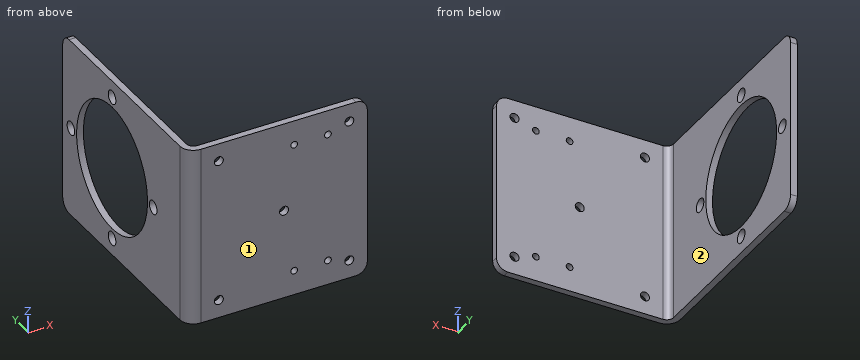
```python
from build123d import *

# Parameters (mm, degrees)
SKETCH1_W                        = 80
SKETCH1_H                        = 98.5
SKETCH1_R                        = 28
BASE_FLANGE1_DEPTH               = 3
F_6_0_6_DIAMETER_HOLE1_D         = 6
CIRPATTERN1_COUNT                = 4
SM_EDGE_FLANGE_1_STRIP_W         = 18
SM_EDGE_FLANGE_1_STRIP_H         = 3
SM_EDGE_FLANGE_1_STRIP_CUT_DEPTH = 80
SM_EDGE_FLANGE_1_DEPTH           = 80
FILLET1_R                        = 5
F_4_0_4_DIAMETER_HOLE4_D         = 4
F_3_0_3_DIAMETER_HOLE2_D         = 3


# Sheet-metal steps are written as plain solids
with BuildPart() as part:
    # Sketch1 → Base-Flange1 (new body)
    with BuildSketch(Plane(origin=(0, 0, 0), x_dir=(0, 0, -1), z_dir=(1, 0, 0))):
        with Locations((40, 49.25)):
            Rectangle(SKETCH1_W, SKETCH1_H)
        with Locations((40, 59.5)):
            Circle(SKETCH1_R, mode=Mode.SUBTRACT)
    extrude(amount=-BASE_FLANGE1_DEPTH)

    # Ø6.0 (6) Diameter Hole1 (through all)
    with Locations(Plane(origin=(0, 0, 0), x_dir=(0, 0, -1), z_dir=(1, 0, 0))):
        with Locations((40, 92)):
            f_6_0_6_diameter_hole1 = Hole(F_6_0_6_DIAMETER_HOLE1_D / 2)

    # CirPattern1: Ø6.0 (6) Diameter Hole1 ×4 about axis
    cirpattern1_axis = Axis((0, 59.5, -40), (1, 0, 0))
    for i in range(1, CIRPATTERN1_COUNT):
        add(f_6_0_6_diameter_hole1.rotate(cirpattern1_axis, i * 360 / CIRPATTERN1_COUNT), mode=Mode.SUBTRACT)

    # 邊線-凸緣1 strip (across the edge) → 邊線-凸緣1 strip cut (cut)
    with BuildSketch(Plane.YX):
        with Locations((-3, -1.5)):
            Rectangle(SM_EDGE_FLANGE_1_STRIP_W, SM_EDGE_FLANGE_1_STRIP_H)
    extrude(amount=SM_EDGE_FLANGE_1_STRIP_CUT_DEPTH, mode=Mode.SUBTRACT)

    # 邊線-凸緣1 section (across the edge) → 邊線-凸緣1 (add)
    with BuildSketch(Plane.YX):
        with BuildLine():
            Line((0, 3), (0, 77))
            Line((0, 77), (3, 77))
            Line((3, 77), (3, 3))
            ThreePointArc((3, 3), (3.878679656, 0.878679656), (6, 0))
            Line((6, 0), (6, -3))
            ThreePointArc((6, -3), (1.757359313, -1.242640687), (0, 3))
        make_face()
    extrude(amount=SM_EDGE_FLANGE_1_DEPTH)

    # Fillet1
    fillet1_edges = [part.edges().sort_by_distance(p)[0] for p in [
        (77, 1.5, 0),
        (77, 1.5, -80),
        (-1.5, 98.5, 0),
        (-1.5, 98.5, -80),
    ]]
    fillet(fillet1_edges, radius=FILLET1_R)

    # Ø4.0 (4) Diameter Hole4 (through all)
    with Locations(Plane(origin=(0, 3, 0), x_dir=(1, 0, 0), z_dir=(0, 1, 0))):
        with Locations((11, 8), (11, 72), (69, 72), (69, 8), (40, 40)):
            Hole(F_4_0_4_DIAMETER_HOLE4_D / 2)

    # Ø3.0 (3) Diameter Hole2 (through all)
    with Locations(Plane(origin=(0, 3, 0), x_dir=(1, 0, 0), z_dir=(0, 1, 0))):
        with Locations((44.5, 11), (59.5, 11)):
            f_3_0_3_diameter_hole2 = Hole(F_3_0_3_DIAMETER_HOLE2_D / 2)

    # Mirror1: Ø3.0 (3) Diameter Hole2 across plane
    add(f_3_0_3_diameter_hole2.mirror(Plane.XY.offset(-40)), mode=Mode.SUBTRACT)


solid = part.part
```
Check sheet for the modelled part. Datum: model origin and axes. Units: mm. Face numbers are marked on the shaded views. A direction names the side the tool comes from. Give positions to 0.01 mm unless a question says otherwise; leave off trailing zeros. Write each loop counter-clockwise with the first axis right and the second up, starting at its lowest first coordinate (ties: lowest second). Pieces come first, ordered by that corner, then holes. Notation, with made-up numbers: (44.5, -28.75) -> (98.5, -28.75) arc R19 ccw to (98.5, -24.75) -> close; hole circle Ø6 at (85.5, 10.25). An arc over 180 degrees is marked (long way). Use CSV: the item, a comma, the result in double quotes. Start each with the question number.
Q1. Cross-section at B-B on z = -40. Enter the section's corners in (x, y).
Q2. Cross-section at D-D on x = 11. Enter the section's corners in (y, z), and give its area (3 significant figures).
Q3. Scan lines: line 1 along Z through (x, y) = (11, 1); line 2 along X through (y, z) = (1, -11); line 3 along X through (y, z) = (2, -69). Record each from-to range of solid material in increasing order.
Q4. Cross-section at C-C on z = -27. Enter the section's corners in (x, y), and give its area (3 significant figures).
Q5. Cross-section at A-A on x = 44.5. Enter the section's corners in (y, z), and give its area (3 significant figures).
Q6. Tool access check on the marked faces 1 and 2. Record the directions out of +Z, -Z, +X, -X, +Y, -Y that give a thin tool (end or side, any length) a straight path to the whole face; none if there is none.
Q7. Depth check by flat-ended pin: P1, Ø4.5, axis at x = 11, z = -8, coming from the +Y side; P2, Ø7, axis at y = 59.5, z = -7.5, coming from the +X side; P3, Ø5, axis at y = 27, z = -40, coming from the -X side. Enter the tip coordinate at first touch or a pass-through.
Working result:
1,outline,"(-3, 6) arc R6 ccw to (3, 0) -> (38, 0) -> (38, 3) -> (3, 3) arc R3 cw to (0, 6) -> (0, 24) -> (-3, 24) -> close; (-3, 30) -> (0, 30) -> (0, 31.5) -> (-3, 31.5) -> close; (-3, 87.5) -> (0, 87.5) -> (0, 89) -> (-3, 89) -> close; (-3, 95) -> (0, 95) -> (0, 98.5) -> (-3, 98.5) -> close; (42, 0) -> (77, 0) -> (77, 3) -> (42, 3) -> close"
2,outline,"(0, -80) -> (3, -80) -> (3, -74) -> (0, -74) -> close; (0, -70) -> (3, -70) -> (3, -10) -> (0, -10) -> close; (0, -6) -> (3, -6) -> (3, 0) -> (0, 0) -> close"
2,area,"216 mm^2"
3,line 1,"z = -80 to -74, -70 to -10, -6 to 0"
3,line 2,"x = -0.32 to 43, 46 to 58, 61 to 77"
3,line 3,"x = -1.47 to 43, 46 to 58, 61 to 77"
4,outline,"(-3, 6) arc R6 ccw to (3, 0) -> (77, 0) -> (77, 3) -> (3, 3) arc R3 cw to (0, 6) -> (0, 34.7) -> (-3, 34.7) -> close; (-3, 84.3) -> (0, 84.3) -> (0, 98.5) -> (-3, 98.5) -> close"
4,area,"372 mm^2"
5,outline,"(0, -80) -> (3, -80) -> (3, -70.5) -> (0, -70.5) -> close; (0, -67.5) -> (3, -67.5) -> (3, -12.5) -> (0, -12.5) -> close; (0, -9.5) -> (3, -9.5) -> (3, 0) -> (0, 0) -> close"
5,area,"222 mm^2"
6,face 1,"+Z, -Z, +X, -X, -Y"
6,face 2,"+Z, -Z, +X, +Y"
7,P1,"stops at y = 3"
7,P2,"stops at x = 0"
7,P3,"passes through"
